For this review, take the finished solid that the model builds, in its own axes (mm). A direction names the side the tool comes from. Give positions to 0.01 mm unless a question says otherwise; leave off trailing zeros. Write each loop counter-clockwise with the first axis right and the second up, starting at its lowest first coordinate (ties: lowest second). Pieces come first, ordered by that corner, then holes. Notation, with made-up numbers: (29.25, 75) -> (87.25, 75) arc R19 ccw to (87.25, 92) -> close; hole circle Ø5 at (37.25, 47.5). An arc over 180 degrees is marked (long way). Write item = value, one per line.
```python
from build123d import *

# Parameters (mm, degrees)
SKETCH_1_R      = 1.5
SKETCH_1_R_2    = 10.5
SKETCH_1_R_3    = 5
SKETCH_1_W      = 10
SKETCH_1_H      = 6
EXTRUDE_1_DEPTH = 6


with BuildPart() as part:
    # Эскиз1 → Бобышка-Вытянуть1 (new body)
    with BuildSketch(Plane(origin=(0, 0, 0), x_dir=(1, 0, 0), z_dir=(0, 1, 0))):
        Polygon((90.453646354, -29.775504496), (90.453646354, -18.275504496), (102.453646354, -18.275504496), (102.453646354, -3.275504496), (90.453646354, -3.275504496), (90.453646354, 6.124495504), (84.453646354, 6.124495504), (84.453646354, 14.224495504), (-76.546353646, 14.224495504), (-76.546353646, 6.124495504), (-82.546353646, 6.124495504), (-82.546353646, -3.275504496), (-94.546353646, -3.275504496), (-94.546353646, -18.275504496), (-82.546353646, -18.275504496), (-82.546353646, -29.775504496), align=None)
        with Locations((-26.046353646, -24.775504496)):
            Circle(SKETCH_1_R, mode=Mode.SUBTRACT)
        with Locations((-66.046353646, -10.775504496)):
            Circle(SKETCH_1_R_2, mode=Mode.SUBTRACT)
        with Locations((-26.046353646, 9.224495504)):
            Circle(SKETCH_1_R, mode=Mode.SUBTRACT)
        with Locations((33.953646354, -24.775504496)):
            Circle(SKETCH_1_R, mode=Mode.SUBTRACT)
        with Locations((73.953646354, -10.775504496)):
            Circle(SKETCH_1_R_2, mode=Mode.SUBTRACT)
        with Locations((33.953646354, 9.224495504)):
            Circle(SKETCH_1_R, mode=Mode.SUBTRACT)
        with Locations((3.953646354, -10.775504496)):
            Circle(SKETCH_1_R_3, mode=Mode.SUBTRACT)
        with Locations((-14.046353646, -24.775504496)):
            Rectangle(SKETCH_1_W, SKETCH_1_H, mode=Mode.SUBTRACT)
        with Locations((-38.046353646, -24.775504496)):
            Rectangle(SKETCH_1_W, SKETCH_1_H, mode=Mode.SUBTRACT)
        with Locations((-14.046353646, 9.224495504)):
            Rectangle(SKETCH_1_W, SKETCH_1_H, mode=Mode.SUBTRACT)
        with Locations((-38.046353646, 9.224495504)):
            Rectangle(SKETCH_1_W, SKETCH_1_H, mode=Mode.SUBTRACT)
        with Locations((21.953646354, -24.775504496)):
            Rectangle(SKETCH_1_W, SKETCH_1_H, mode=Mode.SUBTRACT)
        with Locations((45.953646354, -24.775504496)):
            Rectangle(SKETCH_1_W, SKETCH_1_H, mode=Mode.SUBTRACT)
        with Locations((21.953646354, 9.224495504)):
            Rectangle(SKETCH_1_W, SKETCH_1_H, mode=Mode.SUBTRACT)
        with Locations((45.953646354, 9.224495504)):
            Rectangle(SKETCH_1_W, SKETCH_1_H, mode=Mode.SUBTRACT)
    extrude(amount=EXTRUDE_1_DEPTH)


solid = part.part
```
(1) Take a section at A-A (x = -41). Write out the cut boundary in (y, z).
Answers below:
outline = (0, -14.22) -> (6, -14.22) -> (6, -12.22) -> (0, -12.22) -> close; (0, -6.22) -> (6, -6.22) -> (6, 21.78) -> (0, 21.78) -> close; (0, 27.78) -> (6, 27.78) -> (6, 29.78) -> (0, 29.78) -> close
(2) Take a section at D-D (z = -3). Write out the cut boundary in (x, y).
Answers below:
outline = (-82.55, 0) -> (90.45, 0) -> (90.45, 6) -> (-82.55, 6) -> close
(3) To check wall thickness, follow probe 1 along Z at (x, y) = (-41, 0.3); probe 2 along X at (y, z) = (5.2, 4); probe 3 along X at (y, z) = (1.6, 3). State the ranges of each line that lie inside material, in increasing order.
Answers below:
probe_1 = -14.22 to -12.22, -6.22 to 21.78, 27.78 to 29.78
probe_2 = -94.55 to -74.07, -58.02 to 65.93, 81.98 to 102.45
probe_3 = -82.55 to -73.1, -58.99 to 66.9, 81.01 to 90.45
(4) Take a section at C-C (x = -63.5). Write out the cut boundary in (y, z), plus the area to 3 significant figures.
Answers below:
outline = (0, -14.22) -> (6, -14.22) -> (6, 0.59) -> (0, 0.59) -> close; (0, 20.96) -> (6, 20.96) -> (6, 29.78) -> (0, 29.78) -> close
area = 142 mm^2
(5) Take a section at B-B (z = 14). Write out the cut boundary in (x, y), plus the area to 3 significant figures.
Answers below:
outline = (-94.55, 0) -> (-76.04, 0) -> (-76.04, 6) -> (-94.55, 6) -> close; (-56.05, 0) -> (0.13, 0) -> (0.13, 6) -> (-56.05, 6) -> close; (7.77, 0) -> (63.96, 0) -> (63.96, 6) -> (7.77, 6) -> close; (83.95, 0) -> (102.45, 0) -> (102.45, 6) -> (83.95, 6) -> close
area = 896 mm^2
(6) The part is to be moulded in two halves that separate along Z. For faces 1 (the face through (-33.046, 3, 25)), 2 (the face through (97, 3, 3.276)), say which applies: released by +Z, released by -Z, zero draft, split by the parting line, or undercut.
Answers below:
face_1 = undercut
face_2 = released by -Z
(7) Tool access review of faces 3 (the face through (-14, 3, 21.776)), 4 (the face through (-88, 3, 3.276)): name each direction out of +Z, -Z, +X, -X, +Y, -Y from which nothing blocks a thin tool from reaching the whole face with its end or side.
Answers below:
face_3 = +Y, -Y
face_4 = -Z, -X, +Y, -Y
(8) For pin 1 (3 mm diameter, centred on y = 2.5, z = -2, fed in from -X); pin 2 (3 mm diameter, centred on y = 3.5, z = -8.5, fed in from +X); pin 3 (1.8 mm diameter, centred on x = 99, y = 2, fed in from -Z), all flat-tipped, find the tip position at first contact; note any pin that passes through.
Answers below:
pin_1 = -82.55
pin_2 = 84.45
pin_3 = 3.28
